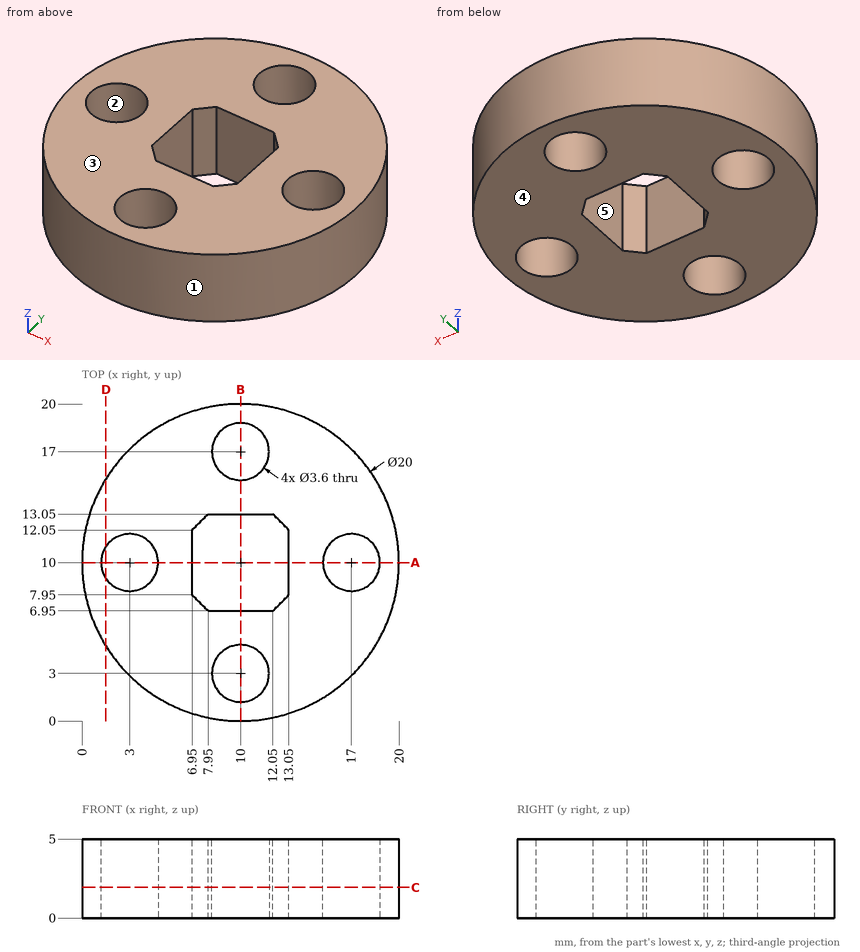
Input: dimensioned drawing with shaded views. Units: mm. Origin: part minimum x, y, z. A direction names the side the tool comes from. Coordinates: 2 decimals unless noted, no trailing zeros. Order: outer loops, then holes, each group sorted by start corner. A loop starts at its lowest first (then second) coordinate and runs counter-clockwise, first axis right, second up. Notation, with made-up numbers: (62.25, 86.25) - (86.25, 86.25) arc R20 cw to (86.25, 105.25) - close; hole circle Ø7 at (38.25, -39). An arc over 180 degrees is marked (long way). One line per item, written item: value.
1) Ray query, line 1 (Y direction, x = 10, z = 1.1); line 2 (X direction, y = 10.5, z = 2.4). Return the intervals inside material, ascending. Write a range as [from, to].
Computed values:
line 1: y = [0, 1.2], [4.8, 6.95], [13.05, 15.2], [18.8, 20]
line 2: x = [0.01, 1.27], [4.73, 6.95], [13.05, 15.27], [18.73, 19.99]
2) Cut plane D-D on x = 1.5. Output: boundary loops of the cut face in (y, z).
Computed values:
outline: (4.73, 0) - (9.01, 0) - (9.01, 5) - (4.73, 5) - close; (10.99, 0) - (15.27, 0) - (15.27, 5) - (10.99, 5) - close
3) Reachability of the marked faces 4 and 5 from +Z, -Z, +X, -X, +Y, -Y: full face, straight path, thin tool, end or side. Return the list, or none.
Computed values:
face 4: -Z, +X, -X, +Y, -Y
face 5: +Z, -Z
4) Mould query, pull axis X, two halves, no side actions, for the marked faces 1, 2 and 3. Classes: released by +X, released by -X, zero draft, split by the parting line, or undercut.
Computed values:
face 1: split by the parting line
face 2: undercut
face 3: zero draft
5) Contact query for flat-ended pins moving along their axis: pin 1 (2 mm diameter, centred on y = 11, z = 3, fed in from +X); pin 2 (3 mm diameter, centred on x = 10, y = 17, fed in from +Z); pin 3 (1.5 mm diameter, centred on y = 14, z = 3, fed in from +X); pin 4 (2 mm diameter, centred on y = 15, z = 3.5, fed in from +X). Output: stop coordinate, or through.
Computed values:
pin 1: stops at x = 20
pin 2: passes through
pin 3: stops at x = 19.46
pin 4: stops at x = 19.17
6) Cut plane C-C on z = 1.95. Output: boundary loops of the cut face in (x, y).
Computed values:
outline: circle Ø20 at (10, 10); hole circle Ø3.6 at (3, 10); hole (6.95, 7.95) - (7.95, 6.95) - (12.05, 6.95) - (13.05, 7.95) - (13.05, 12.05) - (12.05, 13.05) - (7.95, 13.05) - (6.95, 12.05) - close; hole circle Ø3.6 at (10, 3); hole circle Ø3.6 at (10, 17); hole circle Ø3.6 at (17, 10)
7) Cut plane A-A on y = 10. Output: boundary loops of the cut face in (x, z), plus the area to 3 significant figures.
Computed values:
outline: (0, 0) - (1.2, 0) - (1.2, 5) - (0, 5) - close; (4.8, 0) - (6.95, 0) - (6.95, 5) - (4.8, 5) - close; (13.05, 0) - (15.2, 0) - (15.2, 5) - (13.05, 5) - close; (18.8, 0) - (20, 0) - (20, 5) - (18.8, 5) - close
area: 33.5 mm^2
